Study the drawing (mm; zero at the part's minimum x, y, z) and answer. Coordinates: 2 decimals unless noted, no trailing zeros. Loops run counter-clockwise (first coordinate to the right, second up) from the corner with the lowest first, then second, coordinate; pieces in that order, holes last. Notation, with made-up numbers: M 87.25,66 L 99.25,66 A34 cw 99.25,96 Z; hole C -37.75,22 d3. An arc over 180 degrees is marked long. Use one line per item in the form item = value. Start each with the question number.
1. Flat-ended cylindrical pins translate along their axes: pin 1 (2 mm diameter, centred on x = 17.5, z = 4, fed in from +Y); pin 2 (1 mm diameter, centred on x = 29.5, z = 5, fed in from -Y); pin 3 (5 mm diameter, centred on x = 35, y = 10, fed in from +Z). Find the tip coordinate at first contact, or state that the pin passes through.
2. Find the intervals of material crossed by probe 1 along Y at (x, z) = (29.5, 5.75) (1 decimal); probe 2 along Z at (x, y) = (31, 9.5) (1 decimal); probe 3 along Y at (x, z) = (37.5, 7.5), in increasing order. Write a range as [from, to].
3. The part is cut by section A-A (x = 11). Give the vertices of the cut face in (y, z), plus the area to 3 significant figures.
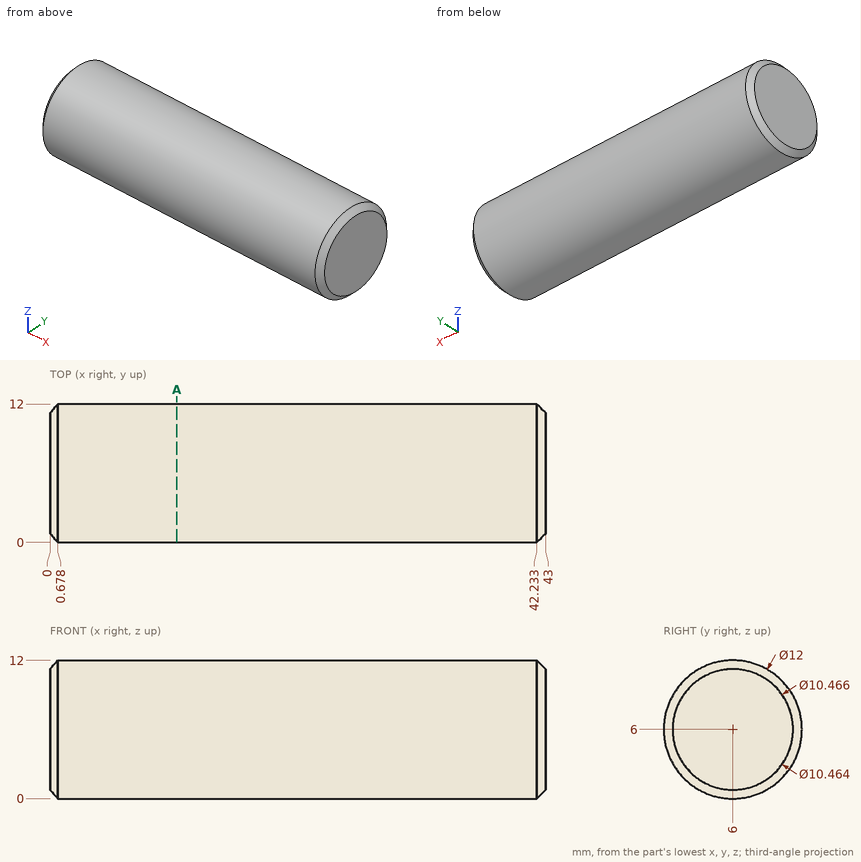
Computed values:
q1.pin_1 = 11.92
q1.pin_2 = 0.02
q1.pin_3 = 11.81
q2.probe_1 = [0, 12]
q2.probe_2 = [1.1, 10.9]
q2.probe_3 = [0.19, 11.81]
q3.outline = C 6,6 d12
q3.area = 113 mm²
